For this review, take the finished solid that the model builds, in its own axes (mm). A direction names the side the tool comes from. Give positions to 0.01 mm unless a question says otherwise; leave off trailing zeros. Use CSV: the item, a comma, the result in double quotes. Start each with the question number.
(1) Tool access review of faces 1 (the face through (317, -27, -4)), 2 (the face through (332, 18, -6)), 3 (the face through (187, 107, -10)): name each direction out of +Z, -Z, +X, -X, +Y, -Y from which nothing blocks a thin tool from reaching the whole face with its end or side.
(2) Draft analysis for pull direction Y (two halves, no side actions). For faces 4 (the face through (401, 30, -2)), 5 (the face through (410, 103, -5)), 6 (the face through (187, -30, -5)), state which applies: pulls with the +Y half, pulls with the -Y half, needs draft (parallel to the pull), parting line crosses it, or undercut.
(3) Clearance check with flat-ended pins moving along their axes: P1, Ø6, axis at x = 65, y = 235, coming from the +Z side; P2, Ø3.5, axis at x = 190, y = 235, coming from the +Z side; P3, Ø4, axis at x = 332.5, y = 189, coming from the -Z side. State where each tip first meets the part, or that it passes through.
(4) Wall thickness on L1, parallel to Y at x = 333.85, z = -8.35; L2, parallel to X at y = 180, z = -8.6; L3, parallel to Y at x = 65, z = -8.15: over which ranges is each line inside the solid? List them lowest first. Write a range as from..to.
```python
from build123d import *

# Parameters (mm, degrees)
SKETCH1_W                      = 440
SKETCH1_H                      = 270
BOSS_EXTRUDE1_DEPTH            = 10
CBORE_FOR_M4_SHCS4_D           = 4.5
CBORE_FOR_M4_SHCS4_DEPTH       = 11.5
CBORE_FOR_M4_SHCS4_CBORE_D     = 8
CBORE_FOR_M4_SHCS4_CBORE_DEPTH = 4
CBORE_FOR_M4_SHCS4_TIP         = 1.351936393
CBORE_FOR_M3_SHCS1_D           = 3.4
CBORE_FOR_M3_SHCS1_CBORE_D     = 6.5
CBORE_FOR_M3_SHCS1_CBORE_DEPTH = 3


with BuildPart() as part:
    # Sketch1 → Boss-Extrude1 (new body)
    with BuildSketch(Plane.XY):
        with Locations((190, 105)):
            Rectangle(SKETCH1_W, SKETCH1_H)
    extrude(amount=-BOSS_EXTRUDE1_DEPTH)

    # Sketch7 → CBORE for M4 SHCS3 (revolve, cut)
    with BuildSketch(Plane(origin=(46.15, 20, -10), x_dir=(0, 1, 0), z_dir=(1, 0, 0))):
        Polygon((0, 0), (0, 12.851936393), (2.25, 11.5), (2.25, 4), (4, 4), (4, 0), align=None)
    cbore_for_m4_shcs3 = revolve(axis=Axis((46.15, 20, -16.35), (0, 0, 1)), mode=Mode.SUBTRACT)

    # Mirror1: CBORE for M4 SHCS3 across plane
    add(cbore_for_m4_shcs3.mirror(Plane(origin=(0, 105, 0), x_dir=(0, 0, 1), z_dir=(0, -1, 0))), mode=Mode.SUBTRACT)

    # Mirror2: CBORE for M4 SHCS3 across plane
    add(cbore_for_m4_shcs3.mirror(Plane.ZY.offset(-190)), mode=Mode.SUBTRACT)

    # Mirror2 copy 1 sketch → Mirror2 copy 1 (revolve, cut)
    with BuildSketch(Plane(origin=(333.85, 190, -10), x_dir=(0, -1, 0), z_dir=(-1, 0, 0))):
        Polygon((0, 0), (0, 12.851936393), (2.25, 11.5), (2.25, 4), (4, 4), (4, 0), align=None)
    revolve(axis=Axis((333.85, 190, -16.35), (0, 0, 1)), mode=Mode.SUBTRACT)

    # CBORE for M4 SHCS4
    with Locations(Plane.XY):
        with Locations((65, 235), (190, 235), (315, 235), (315, -25), (190, -25), (65, -25), (405, 180), (405, 30), (-25, 30), (-25, 180)):
            CounterBoreHole(CBORE_FOR_M4_SHCS4_D / 2, CBORE_FOR_M4_SHCS4_CBORE_D / 2, CBORE_FOR_M4_SHCS4_CBORE_DEPTH, depth=CBORE_FOR_M4_SHCS4_DEPTH)
            with Locations((0, 0, -(CBORE_FOR_M4_SHCS4_DEPTH + CBORE_FOR_M4_SHCS4_TIP / 2))):  # 118° drill point
                Cone(0, CBORE_FOR_M4_SHCS4_D / 2, CBORE_FOR_M4_SHCS4_TIP, mode=Mode.SUBTRACT)

    # Sketch11 → Ø1.0mm Dowel Hole1 (revolve, cut)
    with BuildSketch(Plane(origin=(46.15, 105, 0), x_dir=(0, -1, 0), z_dir=(1, 0, 0))):
        Polygon((0, 0), (0, 5.30043031), (0.5, 5), (0.5, 0), align=None)
    f_1_0mm_dowel_hole1 = revolve(axis=Axis((46.15, 105, 6.35), (0, 0, -1)), mode=Mode.SUBTRACT)

    # Mirror3: Ø1.0mm Dowel Hole1 across plane
    add(f_1_0mm_dowel_hole1.mirror(Plane.ZY.offset(-190)), mode=Mode.SUBTRACT)

    # CBORE for M3 SHCS1 (through all)
    with Locations(Plane.XY):
        with Locations((0, 210)):
            cbore_for_m3_shcs1 = CounterBoreHole(CBORE_FOR_M3_SHCS1_D / 2, CBORE_FOR_M3_SHCS1_CBORE_D / 2, CBORE_FOR_M3_SHCS1_CBORE_DEPTH)

    # Mirror4: CBORE for M3 SHCS1 across plane
    add(cbore_for_m3_shcs1.mirror(Plane.ZY.offset(-190)), mode=Mode.SUBTRACT)


solid = part.part
```
Check result:
1,face 1,"+Z"
1,face 2,"-Z"
1,face 3,"-Z, +X, -X, +Y, -Y"
2,face 4,"undercut"
2,face 5,"needs draft"
2,face 6,"pulls with the -Y half"
3,P1,"stops at z = -4"
3,P2,"passes through"
3,P3,"stops at z = -6"
4,L1,"y = -30..16, 24..186, 194..240"
4,L2,"x = -30..-27.25, -22.75..402.75, 407.25..410"
4,L3,"y = -30..-27.25, -22.75..232.75, 237.25..240"
